```python
from build123d import *

# Parameters (mm, degrees)
F0_R     = 5
F1_DEPTH = 1
F2_R     = 1.25
F3_DEPTH = 6
F4_R     = 1
F5_R     = 0.2


with BuildPart() as f1:
    # F0 (on Top) → F1 (new body)
    with BuildSketch(Plane.XY):
        Circle(F0_R)
    extrude(amount=F1_DEPTH)

    # F2 (on face) → F3 (join)
    with BuildSketch(Plane.XY.offset(1)):
        Circle(F2_R)
    extrude(amount=F3_DEPTH)

    # F4
    f4_edges = [f1.edges().sort_by_distance(p)[0] for p in [
        (-1.25, 0, 7),
    ]]
    fillet(f4_edges, radius=F4_R)

    # F5
    f5_edges = [f1.edges().sort_by_distance(p)[0] for p in [
        (-5, 0, 0),
    ]]
    fillet(f5_edges, radius=F5_R)


solid = f1.part
```
Work out the finished part from the listing and answer in its coordinate system (mm). A direction names the side the tool comes from. Coordinates: 2 decimals unless noted, no trailing zeros. Loops run counter-clockwise (first coordinate to the right, second up) from the corner with the lowest first, then second, coordinate; pieces in that order, holes last.
1) Section A-A (z = 3) is taken. Give the vertices of the cut face in (x, y), plus the area to 3 significant figures.
Results:
outline: circle Ø2.5 at (0, 0)
area: 4.91 mm2
2) Flat-ended cylindrical pins translate along their axes: pin 1 (4 mm diameter, centred on x = -3, z = 1.5, fed in from -Y); pin 2 (3 mm diameter, centred on x = -2, y = 1, fed in from +Z). Find the tip coordinate at first contact, or state that the pin passes through.
Results:
pin 1: stops at y = -4.89
pin 2: stops at z = 6.87
3) For faces 1 (the flat face through (0, 0, 0)), 2 (the flat face through (1, -1, 1)), determine the directions among +Z, -Z, +X, -X, +Y, -Y from which every point of the face is accessible in a straight line to the end or side of a thin tool.
Results:
face 1: -Z, +X, -X, +Y, -Y
face 2: +Z
4) Consider probe 1 along Z at (x, y) = (-0.5, 4); probe 2 along Y at (x, z) = (0.5, 4.5); probe 3 along Y at (x, z) = (-4.5, 0.75). Determine where each line is inside the solid, lowest interval first.
Results:
probe 1: z = 0 to 1
probe 2: y = -1.15 to 1.15
probe 3: y = -2.18 to 2.18
